Build history of the part. All positions in model axes, mm. Face numbers are marked on the shaded views. A direction names the side the tool comes from. Give positions to 0.01 mm unless a question says otherwise; leave off trailing zeros. Order: outer loops, then holes, each group sorted by start corner. A loop starts at its lowest first (then second) coordinate and runs counter-clockwise, first axis right, second up. Notation, with made-up numbers: (-36.5, 49) - (2.5, 49) arc R13 cw to (2.5, 53) - close; hole circle Ø5 at (82, 79.25). An arc over 180 degrees is marked (long way). Answer in a Markdown table with one row per item.
```python
from build123d import *

# Parameters (mm, degrees)
SKETCH1_R           = 10
SKETCH1_R_2         = 3
BOSS_EXTRUDE1_DEPTH = 10
BOSS_EXTRUDE3_START = 5
SKETCH4_R           = 10
BOSS_EXTRUDE3_DEPTH = 5
BOSS_EXTRUDE4_START = 10
SKETCH5_R           = 10
SKETCH5_R_2         = 3
BOSS_EXTRUDE4_DEPTH = 10


with BuildPart() as part:
    # Sketch1 → Boss-Extrude1 (new body)
    with BuildSketch(Plane.XY):
        Circle(SKETCH1_R)
        Circle(SKETCH1_R_2, mode=Mode.SUBTRACT)
    extrude(amount=BOSS_EXTRUDE1_DEPTH)

    # Sketch4 → Boss-Extrude3 (add)
    with BuildSketch(Plane(origin=(0, 0, 0), x_dir=(-1, 0, 0), z_dir=(0, 0, -1)).offset(BOSS_EXTRUDE3_START)):
        Circle(SKETCH4_R)
    extrude(amount=-BOSS_EXTRUDE3_DEPTH)

    # Sketch5 → Boss-Extrude4 (add)
    with BuildSketch(Plane(origin=(0, 0, -5), x_dir=(-1, 0, 0), z_dir=(0, 0, -1)).offset(BOSS_EXTRUDE4_START)):
        Circle(SKETCH5_R)
        with Locations(Location((0, 0, 0), (0, 0, 180))):
            Circle(SKETCH5_R_2, mode=Mode.SUBTRACT)
    extrude(amount=-BOSS_EXTRUDE4_DEPTH)


solid = part.part
```
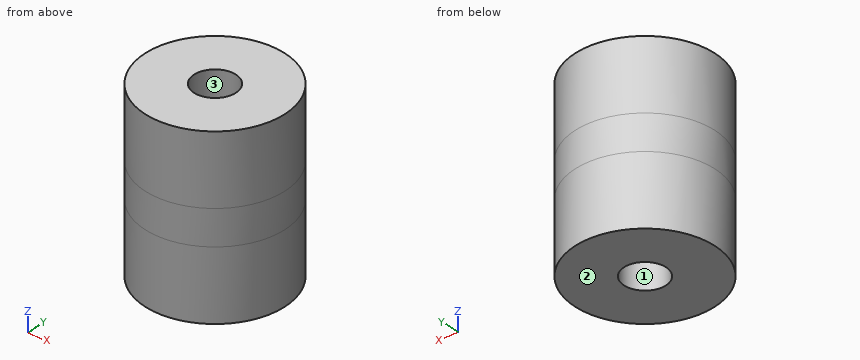
1. Probe line 1 (Y direction, x = 0, z = 5.5); line 2 (Z direction, x = -1.25, y = -1.25); line 3 (X direction, y = 8.25, z = -9). List the from-to ranges inside material, lowest first.
Check result:
| item | result |
|---|---|
| line 1 | y = -10 to -3, 3 to 10 |
| line 2 | z = -5 to 0 |
| line 3 | x = -5.65 to 5.65 |
2. Drop flat-ended pins along their axis: P1, Ø1.8, axis at x = 0, y = 0.5, coming from the -Z side; P2, Ø1.5, axis at y = 5, z = 7, coming from the -X side; P3, Ø12, axis at x = -5.5, z = 0, coming from the +Y side; P4, Ø3, axis at x = -0.5, y = 0, coming from the +Z side. Give the stop position or say it passes through.
Check result:
| item | result |
|---|---|
| P1 | stops at z = -5 |
| P2 | stops at x = -9.05 |
| P3 | stops at y = 10 |
| P4 | stops at z = 0 |
3. Which spindle directions (+Z, -Z, +X, -X, +Y, -Y) get a long thin tool onto all of the face, cutting with end or side? Do the marked faces 1, 2 and 3. Say none if no direction does.
Check result:
| item | result |
|---|---|
| face 1 | -Z |
| face 2 | -Z, +X, -X, +Y, -Y |
| face 3 | +Z |
4. Cut at A-A on y = 0. Write the cut outline in (x, z).
Check result:
| item | result |
|---|---|
| outline | (-10, -15) - (-3, -15) - (-3, -5) - (3, -5) - (3, -15) - (10, -15) - (10, 10) - (3, 10) - (3, 0) - (-3, 0) - (-3, 10) - (-10, 10) - close |
5. Cut at C-C on z = 8.75. Write the cut outline in (x, y).
Check result:
| item | result |
|---|---|
| outline | circle Ø20 at (0, 0); hole circle Ø6 at (0, 0) |
6. Cut at D-D on x = -8. Write the cut outline in (y, z), and give its area (3 significant figures).
Check result:
| item | result |
|---|---|
| outline | (-6, -15) - (6, -15) - (6, 10) - (-6, 10) - close |
| area | 300 mm² |
